Build history of the part. All positions in model axes, mm. A direction names the side the tool comes from. Give positions to 0.01 mm unless a question says otherwise; leave off trailing zeros. Order: outer loops, then holes, each group sorted by start corner. A loop starts at its lowest first (then second) coordinate and runs counter-clockwise, first axis right, second up. Notation, with made-up numbers: M 75.25,17 L 127.25,17 A20 cw 127.25,48 Z; hole C 31,88.25 d4. An arc over 180 degrees is marked long. One line per item, written item: value.
from build123d import *

# Parameters (mm, degrees)
F0_R     = 2.5
F1_DEPTH = 8
F2_R     = 1
F3_DEPTH = 7
F4_R     = 2.5
F5_DEPTH = 2
F6_R     = 6.2
F7_DEPTH = 1


with BuildPart() as f1:
    # F0 (on Top) → F1 (new body)
    with BuildSketch(Plane.XY):
        Circle(F0_R)
    extrude(amount=F1_DEPTH)

    # F2 (on face) → F3 (join)
    with BuildSketch(Plane.XY.offset(8)):
        Circle(F2_R)
    extrude(amount=F3_DEPTH)

    # F4 (on face) → F5 (join)
    with BuildSketch(Plane(origin=(0, 0, 0), x_dir=(1, 0, 0), z_dir=(0, 0, -1))):
        with BuildLine():
            Line((5.5, 7.5), (-5.5, 7.5))
            ThreePointArc((-5.5, 7.5), (-6.9142135624, 6.9142135624), (-7.5, 5.5))
            Line((-7.5, 5.5), (-7.5, -5.5))
            ThreePointArc((-7.5, -5.5), (-6.9142135624, -6.9142135624), (-5.5, -7.5))
            Line((-5.5, -7.5), (5.5, -7.5))
            ThreePointArc((5.5, -7.5), (6.9142135624, -6.9142135624), (7.5, -5.5))
            Line((7.5, -5.5), (7.5, 5.5))
            ThreePointArc((7.5, 5.5), (6.9142135624, 6.9142135624), (5.5, 7.5))
        make_face()
        Circle(F4_R, mode=Mode.SUBTRACT)
        Circle(F4_R)
    extrude(amount=F5_DEPTH)

    # F6 (on face) → F7 (join)
    with BuildSketch(Plane.XY):
        with BuildLine():
            Line((5.5, 7.5), (-5.5, 7.5))
            ThreePointArc((-5.5, 7.5), (-6.9142135624, 6.9142135624), (-7.5, 5.5))
            Line((-7.5, 5.5), (-7.5, -5.5))
            ThreePointArc((-7.5, -5.5), (-6.9142135624, -6.9142135624), (-5.5, -7.5))
            Line((-5.5, -7.5), (5.5, -7.5))
            ThreePointArc((5.5, -7.5), (6.9142135624, -6.9142135624), (7.5, -5.5))
            Line((7.5, -5.5), (7.5, 5.5))
            ThreePointArc((7.5, 5.5), (6.9142135624, 6.9142135624), (5.5, 7.5))
        make_face()
        Circle(F6_R, mode=Mode.SUBTRACT)
    extrude(amount=F7_DEPTH)


solid = f1.part
1) Mould opens along X. For faces 1 (the face through (0, 0, -2)), 2 (the face through (7.5, 0, -1)), 3 (the face through (3, 0, 0)) say: released by +X, released by -X, zero draft, split by the parting line, or undercut.
Check values:
face 1: zero draft
face 2: released by +X
face 3: undercut
2) Saw through at A-A, the plane y = 0. Write the cut outline in (x, z), then the cut area to 3 significant figures.
Check values:
outline: M -7.5,-2 L 7.5,-2 L 7.5,1 L 6.2,1 L 6.2,0 L 2.5,0 L 2.5,8 L 1,8 L 1,15 L -1,15 L -1,8 L -2.5,8 L -2.5,0 L -6.2,0 L -6.2,1 L -7.5,1 Z
area: 86.6 mm^2
3) Pin check, flat tips, straight feed: pin 1 (5 mm diameter, centred on y = -3.5, z = 1.5, fed in from -X); pin 2 (6 mm diameter, centred on y = 1, z = 10, fed in from +X). Stop position of each tip, or through.
Check values:
pin 1: x = -7.5
pin 2: x = 2.5
4) Saw through at C-C, the plane z = 4.5. Write the cut outline in (x, y).
Check values:
outline: C 0,0 d5
5) Saw through at D-D, the plane y = 5.25. Write the cut outline in (x, z), then the cut area to 3 significant figures.
Check values:
outline: M -7.5,-2 L 7.5,-2 L 7.5,1 L 3.3,1 L 3.3,0 L -3.3,0 L -3.3,1 L -7.5,1 Z
area: 38.4 mm^2
6) Tool access for faces 4 (the face through (0, -1, 11)), 5 (the face through (-6.93, -6.9, -0.52)): list every direction of +Z, -Z, +X, -X, +Y, -Y with a clear straight run to the whole face (end or side of a thin tool).
Check values:
face 4: +Z
face 5: +Z, -Z, -X, -Y
7) Drill centre lines: probe 1 along Y at (x, z) = (0, 0.45); probe 2 along Z at (x, y) = (7, -2); probe 3 along Z at (x, y) = (-3, -2.25). Where is each one in solid material? Low to high. Write a range as from..to.
Check values:
probe 1: -7.5..-6.2, -2.5..2.5, 6.2..7.5
probe 2: -2..1
probe 3: -2..0
